Verification items for the finished model (mm, model axes). A direction names the side the tool comes from. Round coordinates to 2 decimals unless told otherwise and drop trailing zeros. Order: outer loops, then holes, each group sorted by start corner. A loop starts at its lowest first (then second) coordinate and runs counter-clockwise, first axis right, second up. Notation, with made-up numbers: (73, 2.5) -> (128, 2.5) arc R14 ccw to (128, 8.5) -> close; hole circle Ø8 at (-24, 58). An arc over 180 degrees is marked (long way). Return JSON: item names as keys, results as strings. Group by question number.
1) Tool access check on faces 4 (the flat face through (-42.605, 46.014, -22.244)), 5 (the flat face through (-37, 29.25, -13)), 6 (the flat face through (-43, 47, -13)), 7 (the flat face through (-43, 40.41, 10)), 8 (the flat face through (-43, 27, -5)). Record the directions out of +Z, -Z, +X, -X, +Y, -Y that give a thin tool (end or side, any length) a straight path to the whole face; none if there is none.
2) Section check B-B on y = 37. Enter the section's corners in (x, z), plus the area to 3 significant figures.
3) Scan lines: L1, parallel to Y at x = -45, z = 17.25; L2, parallel to Y at x = -43.75, z = 15.5; L3, parallel to Y at x = -48, z = 20. Record each from-to range of solid material in increasing order.
4) Section check A-A on x = -45. Enter the section's corners in (y, z).
5) Draft check along Z on faces 1 (the flat face through (-43, 36, -23.258)), 2 (the cylindrical face through (-46.69, -23.42, 18.34)), 3 (the flat face through (-39, 41, -10)). Enter one of: pulls with the +Z half, pulls with the -Z half, needs draft (parallel to the pull), parting line crosses it, or undercut.
6) Depth check by flat-ended pin: pin 1 (5.5 mm diameter, centred on x = -45, y = -22.125, fed in from -Z); pin 2 (6 mm diameter, centred on y = 37, z = -13.26, fed in from -X); pin 3 (4.5 mm diameter, centred on y = 34, z = -15, fed in from +X); pin 4 (4 mm diameter, centred on x = -37, z = -11.5, fed in from -Y). Enter the tip coordinate at first touch or a pass-through.
7) Section check D-D on x = -41.25. Enter the section's corners in (y, z), plus the area to 3 significant figures.
8) Section check C-C on z = -16.5. Enter the section's corners in (x, y), plus the area to 3 significant figures.
```python
from build123d import *

# Parameters (mm, degrees)
SKETCH1_W           = 15
SKETCH1_H           = 54
SKETCH1_R           = 2.1303
BOSS_EXTRUDE1_DEPTH = 10
SKETCH2_W           = 20
SKETCH2_H           = 20
SKETCH2_R           = 5
BOSS_EXTRUDE2_DEPTH = 15
SKETCH5_W           = 26.664475469
SKETCH5_H           = 13.40994033
BOSS_EXTRUDE3_DEPTH = 15
SKETCH3_W           = 16
SKETCH3_H           = 15.5
CUT_EXTRUDE2_DEPTH  = 4
CHAMFER1_SIZE       = 2
CHAMFER2_SIZE       = 2


with BuildPart() as part:
    # Sketch1 → Boss-Extrude1 (new body)
    with BuildSketch(Plane.XY.offset(13.406799166)):
        with Locations((-42.5, 0)):
            Rectangle(SKETCH1_W, SKETCH1_H)
        with Locations((-45, -22.125)):
            Circle(SKETCH1_R, mode=Mode.SUBTRACT)
        with Locations((-45, 22.125)):
            Circle(SKETCH1_R, mode=Mode.SUBTRACT)
    extrude(amount=BOSS_EXTRUDE1_DEPTH)



with BuildPart() as body_2:
    # Sketch2 → Boss-Extrude2 (new body)
    with BuildSketch(Plane.ZY.offset(50)):
        with Locations((-13.257676303, 37)):
            Rectangle(SKETCH2_W, SKETCH2_H)
        with Locations((-13.257676303, 37)):
            Circle(SKETCH2_R, mode=Mode.SUBTRACT)
    extrude(amount=-BOSS_EXTRUDE2_DEPTH)


with BuildPart() as part_1:
    add(part.part)

    add(body_2.part)  # Boss-Extrude3 merges body 2
    # Sketch5 → Boss-Extrude3 (add)
    with BuildSketch(Plane.ZY.offset(50)):
        with Locations((10.074561432, 33.704970165)):
            Rectangle(SKETCH5_W, SKETCH5_H)
    extrude(amount=-BOSS_EXTRUDE3_DEPTH)

    # Sketch3 → Cut-Extrude2 (cut)
    with BuildSketch(Plane(origin=(-35, 0, 0), x_dir=(0, 0, -1), z_dir=(1, 0, 0))):
        with Locations((13.257676303, 37)):
            Rectangle(SKETCH3_W, SKETCH3_H)
    extrude(amount=-CUT_EXTRUDE2_DEPTH, mode=Mode.SUBTRACT)

    # Chamfer1
    chamfer1_edges = [part_1.edges().sort_by_distance(p)[0] for p in [
        (-42.5, 47, -3.257676303),
        (-42.5, 47, -23.257676303),
    ]]
    chamfer(chamfer1_edges, length=CHAMFER1_SIZE)

    # Chamfer2
    chamfer2_edges = [part_1.edges().sort_by_distance(p)[0] for p in [
        (-42.5, 40.40994033, -3.257676303),
        (-42.5, 40.40994033, 23.406799166),
    ]]
    chamfer(chamfer2_edges, length=CHAMFER2_SIZE)


solid = part_1.part
```
Check result:
{
 "1": {"face 4": "-Z, +X, -X, +Y", "face 5": "+X", "face 6": "+Z, -Z, +X, -X, +Y", "face 7": "+Z, +X, -X, +Y", "face 8": "-Z, +X, -X, -Y"},
 "2": {"outline": "(-50, -23.26) -> (-35, -23.26) -> (-35, -21.26) -> (-39, -21.26) -> (-39, -18.26) -> (-50, -18.26) -> close; (-50, -8.26) -> (-39, -8.26) -> (-39, -5.26) -> (-35, -5.26) -> (-35, 23.41) -> (-50, 23.41) -> close", "area": "526 mm^2"},
 "3": {"L1": "-27 to -24.26, -19.99 to 19.99, 24.26 to 40.41", "L2": "-27 to -23.85, -20.4 to 20.4, 23.85 to 40.41", "L3": "-27 to 40.41"},
 "4": {"outline": "(-27, 13.41) -> (-24.26, 13.41) -> (-24.26, 23.41) -> (-27, 23.41) -> close; (-19.99, 13.41) -> (19.99, 13.41) -> (19.99, 23.41) -> (-19.99, 23.41) -> close; (24.26, 13.41) -> (27, 13.41) -> (27, -23.26) -> (45, -23.26) -> (47, -21.26) -> (47, -5.26) -> (45, -3.26) -> (42.41, -3.26) -> (40.41, -1.26) -> (40.41, 21.41) -> (38.41, 23.41) -> (24.26, 23.41) -> close; hole circle Ø10 at (37, -13.26)"},
 "5": {"face 1": "pulls with the -Z half", "face 2": "needs draft", "face 3": "undercut"},
 "6": {"pin 1": "z = 13.41", "pin 2": "through", "pin 3": "x = -39", "pin 4": "y = 27"},
 "7": {"outline": "(-27, 13.41) -> (27, 13.41) -> (27, -23.26) -> (45, -23.26) -> (47, -21.26) -> (47, -5.26) -> (45, -3.26) -> (42.41, -3.26) -> (40.41, -1.26) -> (40.41, 21.41) -> (38.41, 23.41) -> (-27, 23.41) -> close; hole circle Ø10 at (37, -13.26)", "area": "1,220 mm^2"},
 "8": {"outline": "(-50, 27) -> (-35, 27) -> (-35, 29.25) -> (-39, 29.25) -> (-39, 33.19) -> (-50, 33.19) -> close; (-50, 40.81) -> (-39, 40.81) -> (-39, 44.75) -> (-35, 44.75) -> (-35, 47) -> (-50, 47) -> close", "area": "154 mm^2"}
}
